Input: dimensioned drawing with shaded views. Units: mm. Origin: part minimum x, y, z. A direction names the side the tool comes from. Coordinates: 2 decimals unless noted, no trailing zeros. Write each loop counter-clockwise with the first axis right and the second up, starting at its lowest first coordinate (ties: lowest second). Pieces come first, ordered by that corner, then holes. Notation, with made-up numbers: M 50,56 L 60,56 A21 ccw 60,60 Z; hole C 84.25,5 d6. An arc over 180 degrees is marked long. Use one line per item in the form item = value.
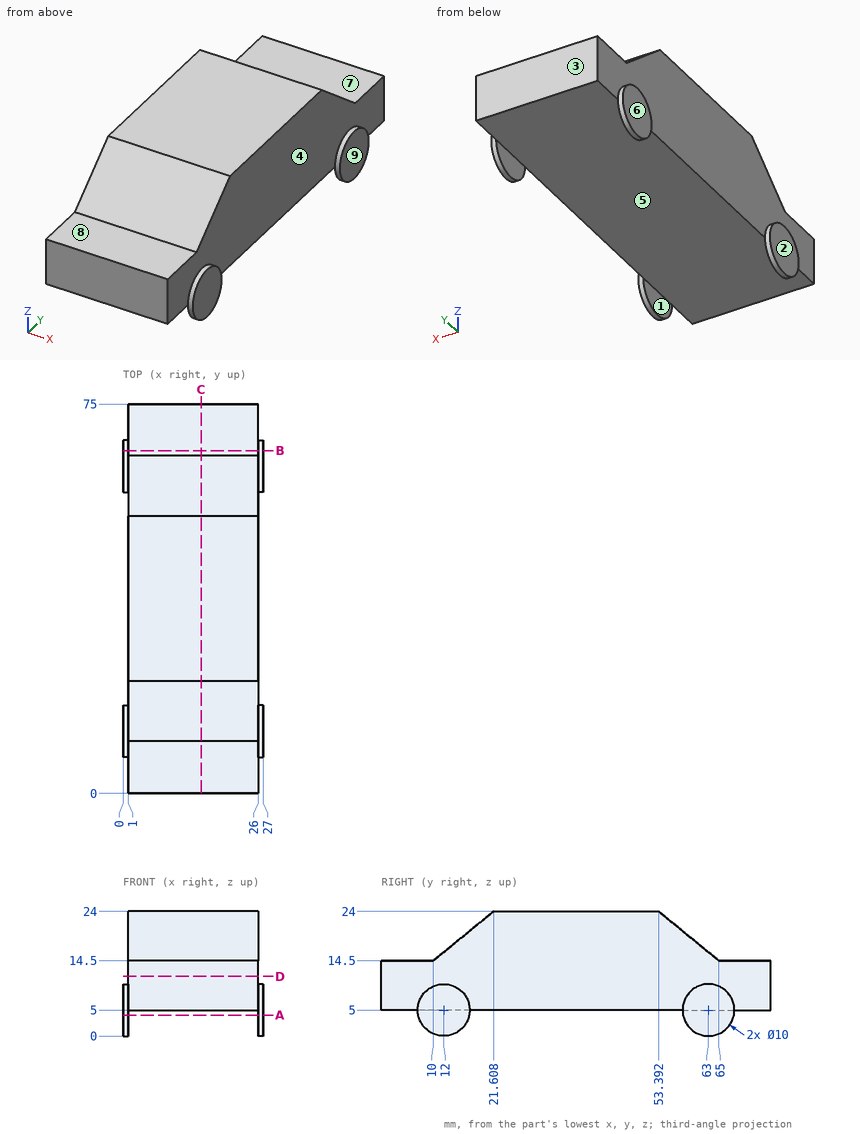
(1) Section query B-B on y = 66. Return the cut outline in (x, z), plus the area to 4 significant figures.
Computed:
outline = M 0,1 L 1,1 L 1,5 L 26,5 L 26,1 L 27,1 L 27,9 L 26,9 L 26,14.5 L 1,14.5 L 1,9 L 0,9 Z
area = 253.5 mm^2
(2) Section query A-A on z = 4. Return the cut outline in (x, y).
Computed:
outline = M 0,7.1 L 1,7.1 L 1,16.9 L 0,16.9 Z; M 0,58.1 L 1,58.1 L 1,67.9 L 0,67.9 Z; M 26,7.1 L 27,7.1 L 27,16.9 L 26,16.9 Z; M 26,58.1 L 27,58.1 L 27,67.9 L 26,67.9 Z
(3) Line query: probe 1 along X at (y, z) = (47.5, 5.5); probe 2 along Z at (x, y) = (22.25, 65.5); probe 3 along Z at (x, y) = (3.25, 24.5). Output: solid intervals per line, ascending.
Computed:
probe_1 = 1 to 26
probe_2 = 5 to 14.5
probe_3 = 5 to 24
(4) Section query D-D on z = 11.5. Return the cut outline in (x, y).
Computed:
outline = M 1,0 L 26,0 L 26,75 L 1,75 Z
(5) Section query C-C on x = 15. Return the cut outline in (y, z), plus the area to 3 significant figures.
Computed:
outline = M 0,5 L 75,5 L 75,14.5 L 65,14.5 L 53.39,24 L 21.61,24 L 10,14.5 L 0,14.5 Z
area = 1,120 mm^2
(6) Pull-direction query (X, two-part tool) for the marked faces 1, 2, 3 and 4; classes: pulls with the +X half, pulls with the -X half, needs draft (parallel to the pull), parting line crosses it, or undercut.
Computed:
face_1 = undercut
face_2 = pulls with the -X half
face_3 = needs draft
face_4 = pulls with the +X half
(7) Set-up query: the marked faces 5, 6, 7, 8 and 9. Return all of +Z, -Z, +X, -X, +Y, -Y with unobstructed straight access to the full face (end or side cutting, diameter ignored); none if empty.
Computed:
face_5 = -Z, +Y, -Y
face_6 = +Z, -Z, -X, +Y, -Y
face_7 = +Z, +X, -X, +Y
face_8 = +Z, +X, -X, -Y
face_9 = +Z, -Z, +X, +Y, -Y
(8) First-contact query: pin 1 Ø10 at (x, y) = (12, 38.5) entering from -Z; pin 2 Ø1 at (x, z) = (6, 9.5) entering from -Y; pin 3 Ø1 at (y, z) = (43, 6) entering from +X; pin 4 Ø3 at (x, y) = (15, 3.5) entering from +Z. Flat tips, straight axial feed; report the tip coordinate or a pass-through.
Computed:
pin_1 = 5
pin_2 = 0
pin_3 = 26
pin_4 = 14.5
